Design review of the part built by this model. Coordinates are the model's own, in mm. A direction names the side the tool comes from. Give positions to 0.01 mm unless a question says otherwise; leave off trailing zeros. Loops run counter-clockwise (first coordinate to the right, second up) from the corner with the lowest first, then second, coordinate; pieces in that order, holes last. Notation, with made-up numbers: M -0.75,88.25 L 30.25,88.25 A20 ccw 30.25,94.25 Z; hole C 34,-8 d5. An arc over 180 degrees is marked long. Use a Markdown table: item, result. Add a question column.
(1) For probe 1 along Y at (x, z) = (-11.8, -85); probe 2 along Z at (x, y) = (-15, 44); probe 3 along Z at (x, y) = (-12.75, 33), list the stretches that pass through material, from the lowest coordinate up.
(2) Insertion check: pin 1 Ø8 at (y, z) = (19, -28) entering from -X; pin 2 Ø1.2 at (x, z) = (-15.5, -50.5) entering from +Y; pin 3 Ø3.5 at (x, z) = (-15, -50) entering from -Y. Each pin has a flat end and moves straight along its axis. Give the tip position at first contact, or say it passes through.
(3) Add section A-A, the plane z = -30. Give the boundary of the cut face in (x, y), then the cut area to 4 significant figures.
(4) Add section D-D, the plane y = 47.5. Give the boundary of the cut face in (x, z), then the cut area to 3 significant figures.
(5) Add section C-C, the plane z = -85. Give the boundary of the cut face in (x, y), then the cut area to 3 significant figures.
(6) For faces 5 (the face through (-15, 26, -57)), 6 (the face through (-15, 15, -10)), 7 (the face through (-16.686, 42.395, -51.075)), list the 3-axis set-ups (+Z, -Z, +X, -X, +Y, -Y) from which the entire face can be reached by the end or side of a thin tool; tool diameter is ignored.
(7) Add section B-B, the plane y = 33. Give the boundary of the cut face in (x, z), then the cut area to 3 significant figures.
(8) Draft analysis for pull direction Y (two halves, no side actions). For faces 1 (the face through (-15, 25, -6)), 2 (the face through (-15, 35, -50)), 3 (the face through (-12.014, 19.217, -76.327)), 4 (the face through (-12, 18, -92)), state which applies: pulls with the +Y half, pulls with the -Y half, needs draft (parallel to the pull), parting line crosses it, or undercut.
```python
from build123d import *

# Parameters (mm, degrees)
ESQUISSE1_W             = 8
ESQUISSE1_H             = 107
BOSS_EXTRU_1_DEPTH      = 50
ESQUISSE4_R             = 1.8
ENL_V_MAT_EXTRU_2_DEPTH = 10
ESQUISSE4_3_R           = 13.4
ESQUISSE4_3_R_2         = 1.8
ESQUISSE4_3_R_3         = 7
ENL_V_MAT_EXTRU_3_DEPTH = 6
ESQUISSE4_4_R           = 7
ENL_V_MAT_EXTRU_4_DEPTH = 10
ENL_V_MAT_EXTRU_5_DEPTH = 10
ESQUISSE26_R            = 7.95
ENL_V_MAT_EXTRU_6_DEPTH = 10
ESQUISSE24_R            = 8.2
ESQUISSE24_R_2          = 5.5
BOSS_EXTRU_6_DEPTH      = 3
ESQUISSE29_R            = 2
ENL_V_MAT_EXTRU_7_DEPTH = 15
ENL_V_START             = -15
ESQUISSE30_R            = 2
ENL_V_MAT_EXTRU_8_DEPTH = 15


with BuildPart() as part:
    # Esquisse1 → Boss.-Extru.1 (new body)
    with BuildSketch(Plane(origin=(0, 0, 0), x_dir=(1, 0, 0), z_dir=(0, 1, 0))):
        with Locations((-15, 59.5)):
            Rectangle(ESQUISSE1_W, ESQUISSE1_H)
    extrude(amount=BOSS_EXTRU_1_DEPTH)

    # Esquisse4 → Enl_v. mat.-Extru.2 (cut)
    with BuildSketch(Plane.ZY.offset(19)):
        with Locations((-95, 18)):
            Circle(ESQUISSE4_R)
        with Locations((-85, 28)):
            Circle(ESQUISSE4_R)
        with Locations((-85, 8)):
            Circle(ESQUISSE4_R)
        with Locations((-75, 18)):
            Circle(ESQUISSE4_R)
    extrude(amount=-ENL_V_MAT_EXTRU_2_DEPTH, mode=Mode.SUBTRACT)

    # Esquisse4_3 → Enl_v. mat.-Extru.3 (cut)
    with BuildSketch(Plane.ZY.offset(19)):
        with Locations((-85, 18)):
            Circle(ESQUISSE4_3_R)
        with Locations((-95, 18)):
            Circle(ESQUISSE4_3_R_2, mode=Mode.SUBTRACT)
        with Locations((-85, 28)):
            Circle(ESQUISSE4_3_R_2, mode=Mode.SUBTRACT)
        with Locations((-75, 18)):
            Circle(ESQUISSE4_3_R_2, mode=Mode.SUBTRACT)
        with Locations((-85, 8)):
            Circle(ESQUISSE4_3_R_2, mode=Mode.SUBTRACT)
        with Locations((-85, 18)):
            Circle(ESQUISSE4_3_R_3, mode=Mode.SUBTRACT)
    extrude(amount=-ENL_V_MAT_EXTRU_3_DEPTH, mode=Mode.SUBTRACT)

    # Esquisse4_4 → Enl_v. mat.-Extru.4 (cut)
    with BuildSketch(Plane.ZY.offset(19)):
        with Locations((-85, 18)):
            Circle(ESQUISSE4_4_R)
    extrude(amount=-ENL_V_MAT_EXTRU_4_DEPTH, mode=Mode.SUBTRACT)

    # Esquisse9 → Enl_v. mat.-Extru.5 (cut)
    with BuildSketch(Plane.ZY.offset(19)):
        with BuildLine():
            ThreePointArc((-57, 39), (-60, 42), (-63, 39))
            Line((-63, 39), (-63, 13))
            ThreePointArc((-63, 13), (-60, 10), (-57, 13))
            Line((-57, 13), (-57, 39))
        make_face()
    extrude(amount=-ENL_V_MAT_EXTRU_5_DEPTH, mode=Mode.SUBTRACT)

    # Esquisse26 → Enl_v. mat.-Extru.6 (cut)
    with BuildSketch(Plane(origin=(-11, 0, 0), x_dir=(0, 0, -1), z_dir=(1, 0, 0))):
        with Locations((30, 18)):
            Circle(ESQUISSE26_R)
    extrude(amount=-ENL_V_MAT_EXTRU_6_DEPTH, mode=Mode.SUBTRACT)

    # Esquisse24 → Boss.-Extru.6 (add)
    with BuildSketch(Plane(origin=(-11, 0, 0), x_dir=(0, 0, -1), z_dir=(1, 0, 0))):
        with Locations((30, 18)):
            Circle(ESQUISSE24_R)
        with Locations((30, 18)):
            Circle(ESQUISSE24_R_2, mode=Mode.SUBTRACT)
    extrude(amount=-BOSS_EXTRU_6_DEPTH)

    # Esquisse29 → Enl_v. mat.-Extru.7 (cut)
    with BuildSketch(Plane.XZ):
        with Locations(Location((-15, -109, 0), (0, 0, 270))):
            Circle(ESQUISSE29_R)
        with Locations(Location((-15, -10, 0), (0, 0, 270))):
            Circle(ESQUISSE29_R)
        with Locations(Location((-15, -50, 0), (0, 0, 270))):
            Circle(ESQUISSE29_R)
    extrude(amount=-ENL_V_MAT_EXTRU_7_DEPTH, mode=Mode.SUBTRACT)

    # Esquisse30 → Enl_v. mat.-Extru.8 (cut)
    with BuildSketch(Plane(origin=(0, 50, 0), x_dir=(1, 0, 0), z_dir=(0, 1, 0)).offset(ENL_V_START)):
        with Locations(Location((-15, 10, 0), (0, 0, 90))):
            Circle(ESQUISSE30_R)
        with Locations(Location((-15, 50, 0), (0, 0, 90))):
            Circle(ESQUISSE30_R)
    extrude(amount=ENL_V_MAT_EXTRU_8_DEPTH, mode=Mode.SUBTRACT)


solid = part.part
```
Established:
| question | item | result |
|---|---|---|
| 1 | probe 1 | 0 to 6.2, 9.8 to 11, 25 to 26.2, 29.8 to 50 |
| 1 | probe 2 | -113 to -52, -48 to -12, -8 to -6 |
| 1 | probe 3 | -113 to -63, -57 to -6 |
| 2 | pin 1 | x = -14 |
| 2 | pin 2 | y = 35 |
| 2 | pin 3 | y = 15 |
| 3 | outline | M -19,0 L -11,0 L -11,12.5 L -14,12.5 L -14,10.05 L -19,10.05 Z; M -19,25.95 L -14,25.95 L -14,23.5 L -11,23.5 L -11,50 L -19,50 Z |
| 3 | area | 287.5 mm^2 |
| 4 | outline | M -19,-113 L -11,-113 L -11,-6 L -19,-6 Z; hole C -15,-50 d4; hole C -15,-10 d4 |
| 4 | area | 831 mm^2 |
| 5 | outline | M -19,0 L -11,0 L -11,6.2 L -13,6.2 L -13,4.6 L -19,4.6 Z; M -19,31.4 L -13,31.4 L -13,29.8 L -11,29.8 L -11,50 L -19,50 Z; M -13,9.8 L -11,9.8 L -11,11 L -13,11 Z; M -13,25 L -11,25 L -11,26.2 L -13,26.2 Z |
| 5 | area | 197 mm^2 |
| 6 | face 5 | +X, -X |
| 6 | face 6 | -Y |
| 6 | face 7 | +Y |
| 7 | outline | M -19,-113 L -11,-113 L -11,-63 L -19,-63 Z; M -19,-57 L -11,-57 L -11,-6 L -19,-6 Z |
| 7 | area | 808 mm^2 |
| 8 | face 1 | needs draft |
| 8 | face 2 | pulls with the +Y half |
| 8 | face 3 | undercut |
| 8 | face 4 | undercut |
